from build123d import *

# Parameters (mm, degrees)
F1_DEPTH = 25.4
F3_D     = 10.71626
F3_DEPTH = 18.5615384615
F3_TIP   = 3.2194893086
F5_D     = 10.71626
F5_DEPTH = 18.561558
F5_TIP   = 3.2194893086


with BuildPart() as f1:
    # F0 (on Right) → F1 (new body)
    with BuildSketch(Plane.YZ):
        Polygon((0, 355.6), (0, 0), (177.8, 0), (177.8, 25.4), (25.4, 355.6), align=None)
    extrude(amount=-F1_DEPTH)

    # F3
    with Locations(Plane.XZ):
        with Locations((-12.7, 317.5), (-12.7, 203.2)):
            Hole(F3_D / 2, depth=F3_DEPTH)
            with Locations((0, 0, -(F3_DEPTH + F3_TIP / 2))):  # 118° drill point
                Cone(0, F3_D / 2, F3_TIP, mode=Mode.SUBTRACT)

    # F5
    with Locations(Plane(origin=(0, 0, 0), x_dir=(1, 0, 0), z_dir=(0, 0, -1))):
        with Locations((-12.7, -50.8), (-12.7, -139.7)):
            Hole(F5_D / 2, depth=F5_DEPTH)
            with Locations((0, 0, -(F5_DEPTH + F5_TIP / 2))):  # 118° drill point
                Cone(0, F5_D / 2, F5_TIP, mode=Mode.SUBTRACT)


solid = f1.part
Source: CAD feature listing. Evaluate the final solid. Frame: model axes, mm. A direction names the side the tool comes from. Round coordinates to 2 decimals unless told otherwise and drop trailing zeros. Loops run counter-clockwise (first coordinate to the right, second up) from the corner with the lowest first, then second, coordinate; pieces in that order, holes last. Notation, with made-up numbers: (65, 2) -> (100, 2) arc R15 cw to (100, 17) -> close; hole circle Ø2 at (-33, -29.5). An arc over 180 degrees is marked (long way). Answer as a JSON object with one key per item and string values. Group by question number.
Q1. Section query A-A (x = -22). Output: boundary loops of the cut face in (y, z).
Q2. Mould query, pull axis X, two halves, no side actions, for faces 1 (the flat face through (0, 68, 141)), 2 (the conical face through (-12.9, 140.61, 21.22)), 3 (the flat face through (-12.522, 102.667, 188.189)), 4 (the flat face through (-25.4, 68, 141)). Classes: pulls with the +X half, pulls with the -X half, needs draft (parallel to the pull), parting line crosses it, or undercut.
Q3. Section query C-C (y = 125). Output: boundary loops of the cut face in (x, z).
Q4. Section query B-B (z = 119). Output: boundary loops of the cut face in (x, y).
Q5. Contact query for flat-ended pins moving along their axis: P1, Ø4, axis at x = -3, z = 273, coming from the +Y side; P2, Ø14, axis at x = -12.7, y = 50.8, coming from the +Z side; P3, Ø9.5, axis at x = -12.7, z = 203.2, coming from the +Y side. Output: stop coordinate, or through.
Q6. Access query for faces 5 (the cylindrical face through (-11.54, 144.93, 9.41)), 6 (the flat face through (-13, 177.8, 13)), 7 (the cylindrical face through (-11.54, 9.41, 312.27)). Directions: +Z, -Z, +X, -X, +Y, -Y. A direction counts if a zero-diameter tool reaches every point of the face in a straight line with its end or side. Return the directions, or none.
Q7. Ray query, line 1 (Z direction, x = -12.7, y = 4.5); line 2 (Y direction, x = -12.7, z = 7.25); line 3 (X direction, y = 6.5, z = 317.5). Return the intervals inside material, ascending. Write a range as from..to.
Completed:
{
 "1": {"outline": "(0, 0) -> (177.8, 0) -> (177.8, 25.4) -> (25.4, 355.6) -> (0, 355.6) -> close"},
 "2": {"face 1": "pulls with the +X half", "face 2": "undercut", "face 3": "needs draft", "face 4": "pulls with the -X half"},
 "3": {"outline": "(-25.4, 0) -> (0, 0) -> (0, 139.8) -> (-25.4, 139.8) -> close"},
 "4": {"outline": "(-25.4, 0) -> (0, 0) -> (0, 134.6) -> (-25.4, 134.6) -> close"},
 "5": {"P1": "y = 64.45", "P2": "z = 315.73", "P3": "y = 97.93"},
 "6": {"face 5": "-Z", "face 6": "+Z, -Z, +X, -X, +Y", "face 7": "-Y"},
 "7": {"line 1": "0..197.84, 208.56..312.14, 322.86..355.6", "line 2": "0..45.44, 56.16..134.34, 145.06..177.8", "line 3": "-25.4..-18.06, -7.34..0"}
}
